Autodesk Inventor part; units mm, degrees
ref_plane "YZ Plane" through (0, 0, 0) normal (1, 0, 0) x (0, 1, 0)
ref_plane "XZ Plane" through (0, 0, 0) normal (0, 1, 0) x (-1, 0, 0)
ref_plane "XY Plane" through (0, 0, 0) normal (0, 0, 1) x (1, 0, 0)
sketch "Sketch1" plane through (0, 0, 0) normal (1, 0, 0) x (0, 1, 0)
  line L0 (0, 0) -> (0, 201.966)
  circle A0 centre (12.3, 22.683) radius 7.8
  line L1 (0, 0) -> (16.4683, 0)
  circle A1 centre (12.3, 201.966) radius 7.8
  line L2 (0, 0) -> (28.5, 0)
  line L3 (28.5, 0) -> (28.5, 174.8193)
  line L4 (12.3, 22.683) -> (149.7256, 99.4246) construction
  circle A2 centre (149.7256, 99.4246) radius 7.8
  line L5 (28.5, 174.8193) -> (141.0282, 90.7272)
  arc A3 (141.0282, 90.7272) -> (158.423, 108.122) centre (149.7256, 99.4246) ccw
  line L6 (149.7256, 99.4246) -> (158.423, 108.122) construction
  line L7 (149.7256, 99.4246) -> (141.0282, 90.7272) construction
  line L8 (158.423, 108.122) -> (19.517, 211.9262)
  arc A4 (19.517, 211.9262) -> (0, 201.966) centre (12.3, 201.966) ccw
  dimension "d0" = 201.966
  dimension "d1" = 22.683
  dimension "d2" = 12.3
  dimension "d5" = 28.5
  dimension "d6" = 157.401
  dimension "d7" = 119.18
  dimension "d8" = 15.6
  dimension "d10" = 180
  dimension "d11" = 12.3
  dimension "d12" = 12.3
  dimension "d13" = 9.9602
extrude "Extrusion1" add sketch "Sketch1" along normal blind 9
fillet "Fillet1" radius 4 2 edges at (4.5, 28.5, 0) (4.5, 0, 0)
sketch "Sketch2" plane through (9, 0, 0) normal (1, 0, 0) x (0, 0, -1)
  circle A0 centre (-201.966, 12.3) radius 7.8
  circle A1 centre (-201.966, 12.3) radius 3.8
  point P0 (0, 0)
  dimension "d17" = 15.6
  dimension "d18" = 7.6
extrude "Extrusion2" add sketch "Sketch2" against normal blind 9
equation "\"d2\" = altura_hoyo"
equation "\"d6\" = d_entre_ejes"
equation "\"d12\" = d11"
properties part number "Marco_trasero_triciclo" material "Aluminum 6061"
Geometry: final body of the model. Coordinates: model frame, mm. A direction names the side the tool comes from. Give positions to 0.01 mm unless a question says otherwise; leave off trailing zeros. Loops run counter-clockwise (first coordinate to the right, second up) from the corner with the lowest first, then second, coordinate; pieces in that order, holes last. Notation, with made-up numbers: M 23.25,-10.5 L 37.25,-10.5 A12 cw 37.25,-5.5 Z; hole C 87,55.25 d5. An arc over 180 degrees is marked long. Put each result on its own line as item: value.
1) Cut plane C-C, the plane y = 144.5. Return the cut outline in (x, z).
Computed values:
outline: M 0,88.29 L 9,88.29 L 9,93.63 L 0,93.63 Z; M 0,105.22 L 9,105.22 L 9,118.53 L 0,118.53 Z
2) Cut plane A-A, the plane y = 12.3. Return the cut outline in (x, z), plus the area to 3 significant figures.
Computed values:
outline: M 0,0 L 9,0 L 9,14.88 L 0,14.88 Z; M 0,30.48 L 9,30.48 L 9,198.17 L 0,198.17 Z; M 0,205.77 L 9,205.77 L 9,214.27 L 0,214.27 Z
area: 1,720 mm^2
3) First-contact query: P1, Ø5, axis at x = 7, y = 126, coming from the +Z side; P2, Ø1, axis at x = 3.5, y = 39, coming from the -Z side; P3, Ø2, axis at x = 4, z = 186.5, coming from the +Y side; P4, Ø12.5, axis at y = 149.73, z = 99.42, coming from the +X side. Flat tips, straight axial feed; report the tip coordinate or a pass-through.
Computed values:
P1: stops at z = 134.22
P2: stops at z = 166.6
P3: stops at y = 54.88
P4: passes through
4) Cut plane D-D, the plane z = 183. Return the cut outline in (x, y), plus the area to 3 significant figures.
Computed values:
outline: M 0,0 L 9,0 L 9,58.22 L 0,58.22 Z
area: 524 mm^2
5) Material intervals for L1, parallel to Y at x = 6.75, z = 23; L2, parallel to Y at x = 3, z = 105; L3, parallel to Y at x = 1.75, z = 33, sorted ascending. Write a range as from..to.
Computed values:
L1: y = 0..4.51, 20.09..28.5
L2: y = 0..28.5, 121.93..144.27, 155.18..160.69
L3: y = 0..28.5
6) Cut plane B-B, the plane x = 6.5. Return the cut outline in (y, z).
Computed values:
outline: M 0,4 A4 ccw 4,0 L 24.5,0 A4 ccw 28.5,4 L 28.5,174.82 L 141.03,90.73 A12.3 ccw 158.42,108.12 L 19.52,211.93 A12.3 ccw 0,201.97 Z; hole C 12.3,22.68 d15.6; hole C 12.3,201.97 d7.6; hole C 149.73,99.42 d15.6
7) Reachability of faces 4 (the cylindrical face through (4.44, 158.61, 90.92)), 5 (the flat face through (4, 28.5, 88)) from +Z, -Z, +X, -X, +Y, -Y: full face, straight path, thin tool, end or side. Return the list, or none.
Computed values:
face 4: +X, -X
face 5: -Z, +X, -X
8) Mould query, pull axis Z, two halves, no side actions, for faces 1 (the flat face through (9, 27, 108)), 2 (the cylindrical face through (4.563, 12.467, 205.762)), 3 (the cylindrical face through (4.437, 6.541, 212.835)). Classes: released by +Z, released by -Z, zero draft, split by the parting line, or undercut.
Computed values:
face 1: zero draft
face 2: undercut
face 3: released by +Z
